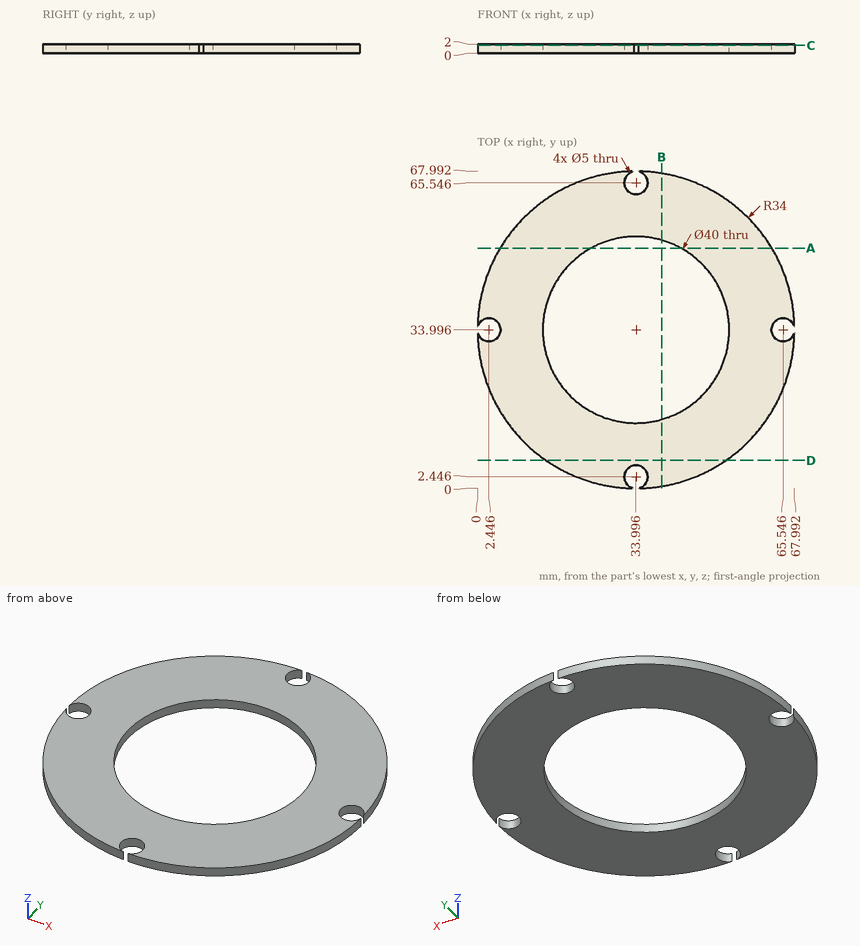
Input: dimensioned drawing with shaded views. Units: mm. Origin: part minimum x, y, z. Give positions to 0.01 mm unless a question says otherwise; leave off trailing zeros. Loops run counter-clockwise (first coordinate to the right, second up) from the corner with the lowest first, then second, coordinate; pieces in that order, holes last. Notation, with made-up numbers: (7.5, -35.5) -> (51.5, -35.5) arc R16 ccw to (51.5, -23.5) -> close; hole circle Ø8 at (67.25, 14). An arc over 180 degrees is marked (long way). Return JSON: item names as keys, results as strings.
Item 1: Pin query (flat end, axial travel): P1, Ø4.5, axis at x = 65.55, y = 34, coming from the +Z side; P2, Ø1, axis at x = 33.5, z = 1, coming from the -Y side. Return the tip coordinate at first contact, or that it passes through.
Filled in:
{"P1": "through", "P2": "y = 0"}
Item 2: Section C-C, the plane z = 1.7. Output: boundary loops of the cut face in (x, y), plus the area to 3 significant figures.
Filled in:
{"outline": "(0, 33.48) arc R34 ccw to (33.48, 0) arc R2.5 cw (long way) to (34.51, 0) arc R34 ccw to (67.99, 33.48) arc R2.5 cw (long way) to (67.99, 34.51) arc R34 ccw to (34.51, 67.99) arc R2.5 cw (long way) to (33.48, 67.99) arc R34 ccw to (0, 34.51) arc R2.5 cw (long way) to start; hole circle Ø40 at (34, 34)", "area": "2,300 mm^2"}
Item 3: Section D-D, the plane y = 6. Output: boundary loops of the cut face in (x, z).
Filled in:
{"outline": "(14.7, 0) -> (53.29, 0) -> (53.29, 2) -> (14.7, 2) -> close"}
Item 4: Line query: line 1 (Y direction, x = 32.5, z = 0.6); line 2 (X direction, y = 39, z = 0.1); line 3 (X direction, y = 43, z = 1.9) (1 decimal). Output: solid intervals per line, ascending.
Filled in:
{"line 1": "0.03 to 0.44, 4.45 to 14.05, 53.94 to 63.54, 67.55 to 67.96", "line 2": "0.37 to 14.63, 53.36 to 67.63", "line 3": "1.2 to 16.1, 51.9 to 66.8"}
Item 5: Section A-A, the plane y = 51.5. Output: boundary loops of the cut face in (x, z), plus the area to 3 significant figures.
Filled in:
{"outline": "(4.85, 0) -> (24.32, 0) -> (24.32, 2) -> (4.85, 2) -> close; (43.67, 0) -> (63.14, 0) -> (63.14, 2) -> (43.67, 2) -> close", "area": "77.9 mm^2"}
Item 6: Section B-B, the plane x = 39.5. Output: boundary loops of the cut face in (y, z), plus the area to 3 significant figures.
Filled in:
{"outline": "(0.44, 0) -> (14.77, 0) -> (14.77, 2) -> (0.44, 2) -> close; (53.22, 0) -> (67.55, 0) -> (67.55, 2) -> (53.22, 2) -> close", "area": "57.3 mm^2"}
